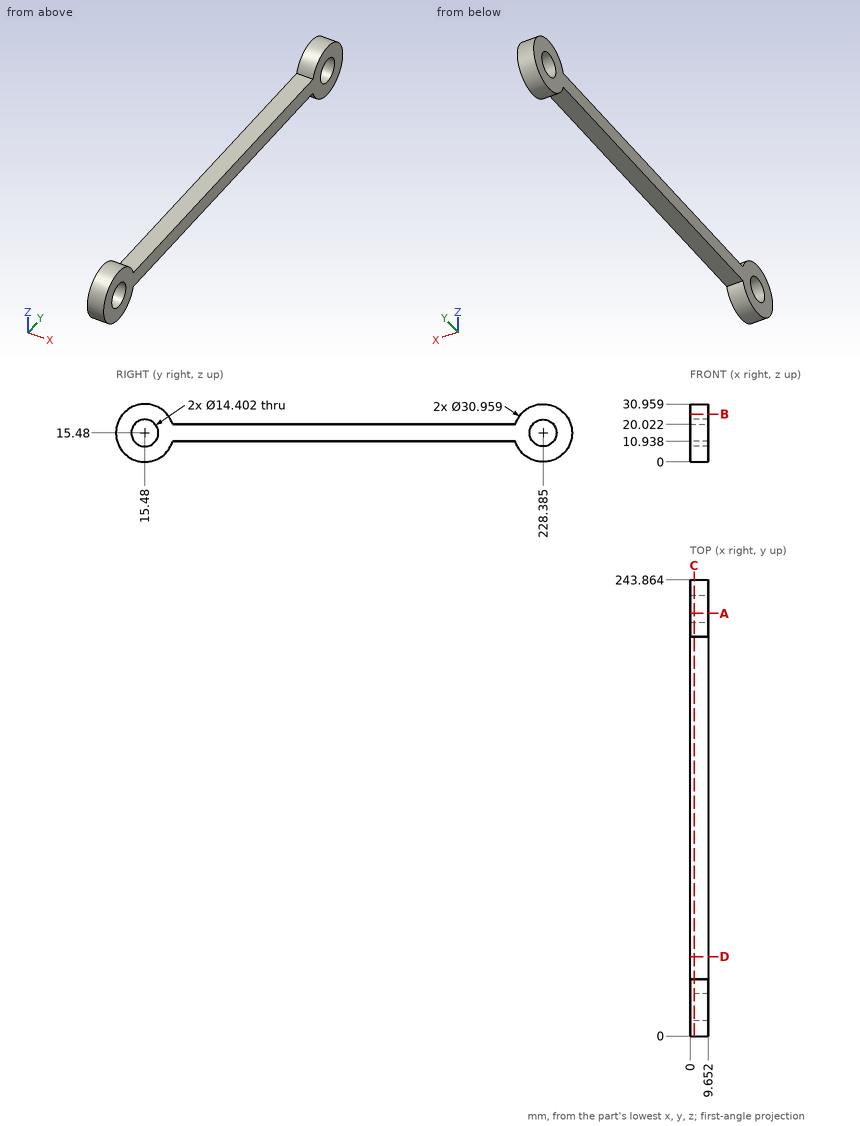
Could you check a few things on this drawing? It's one solid part, dimensions in mm from its lowest x, y, z. Give positions to 0.01 mm unless a question says otherwise; leave off trailing zeros. Order: outer loops, then holes, each group sorted by start corner. A loop starts at its lowest first (then second) coordinate and runs counter-clockwise, first axis right, second up. Notation, with made-up numbers: (8.5, -12.5) -> (56.5, -12.5) arc R17 cw to (56.5, -7.5) -> close; hole circle Ø3 at (-35, 31). An arc over 180 degrees is marked (long way). Answer in a Markdown table with one row per item. Add a question column.
Item 1: Imagine slicing it at A-A (y = 226). List the corners of the cut face in (x, z) for me (1 decimal).
Item 2: Imagine slicing it at C-C (x = 2.25). List the corners of the cut face in (y, z) for me (1 decimal).
Item 3: Imagine slicing it at D-D (y = 42.5). List the corners of the cut face in (x, z) for me.
Item 4: I'm going to push flat-ended pins straight in: P1, Ø2, axis at x = 7.5, y = 174.5, coming from the -Z side; P2, Ø5, axis at x = 5, y = 93, coming from the +Z side; P3, Ø1, axis at x = 3.5, z = 13.5, coming from the +Y side. Where does each tip first touch, or does it pass through?
Item 5: Imagine slicing it at B-B (z = 25.5). List the corners of the cut face in (x, y) for me (1 decimal).
Item 6: Please list where these lines run through material, in increasing order: probe 1 along Y at (x, z) = (4.25, 16) (1 decimal); probe 2 along Z at (x, y) = (7, 118.5); probe 3 along Y at (x, z) = (8, 27) (1 decimal).
Result:
| question | item | result |
|---|---|---|
| 1 | outline | (0, 0.2) -> (9.7, 0.2) -> (9.7, 8.7) -> (0, 8.7) -> close; (0, 22.3) -> (9.7, 22.3) -> (9.7, 30.8) -> (0, 30.8) -> close |
| 2 | outline | (30.3, 10.9) -> (213.6, 10.9) arc R15.5 ccw (long way) to (213.6, 20) -> (30.3, 20) arc R15.5 ccw (long way) to start; hole circle Ø14.4 at (15.5, 15.5); hole circle Ø14.4 at (228.4, 15.5) |
| 3 | outline | (0, 10.94) -> (9.65, 10.94) -> (9.65, 20.02) -> (0, 20.02) -> close |
| 4 | P1 | z = 10.94 |
| 4 | P2 | z = 20.02 |
| 4 | P3 | y = 243.79 |
| 5 | outline | (0, 3.7) -> (9.7, 3.7) -> (9.7, 27.3) -> (0, 27.3) -> close; (0, 216.6) -> (9.7, 216.6) -> (9.7, 240.2) -> (0, 240.2) -> close |
| 6 | probe 1 | 0 to 8.3, 22.7 to 221.2, 235.6 to 243.9 |
| 6 | probe 2 | 10.94 to 20.02 |
| 6 | probe 3 | 5.1 to 25.8, 218 to 238.7 |
